Design review of the part shown in the three views and the two pictorial views. Dimensions are in mm from the part's minimum x, y and z. A direction names the side the tool comes from. Give positions to 0.01 mm unless a question says otherwise; leave off trailing zeros. Loops run counter-clockwise (first coordinate to the right, second up) from the corner with the lowest first, then second, coordinate; pieces in that order, holes last. Notation, with made-up numbers: (67, 24) - (79, 24) arc R26 ccw to (79, 40) - close; hole circle Ø1 at (43, 42.25). An arc over 180 degrees is marked (long way). Answer as a JSON object with one key per item and string values.
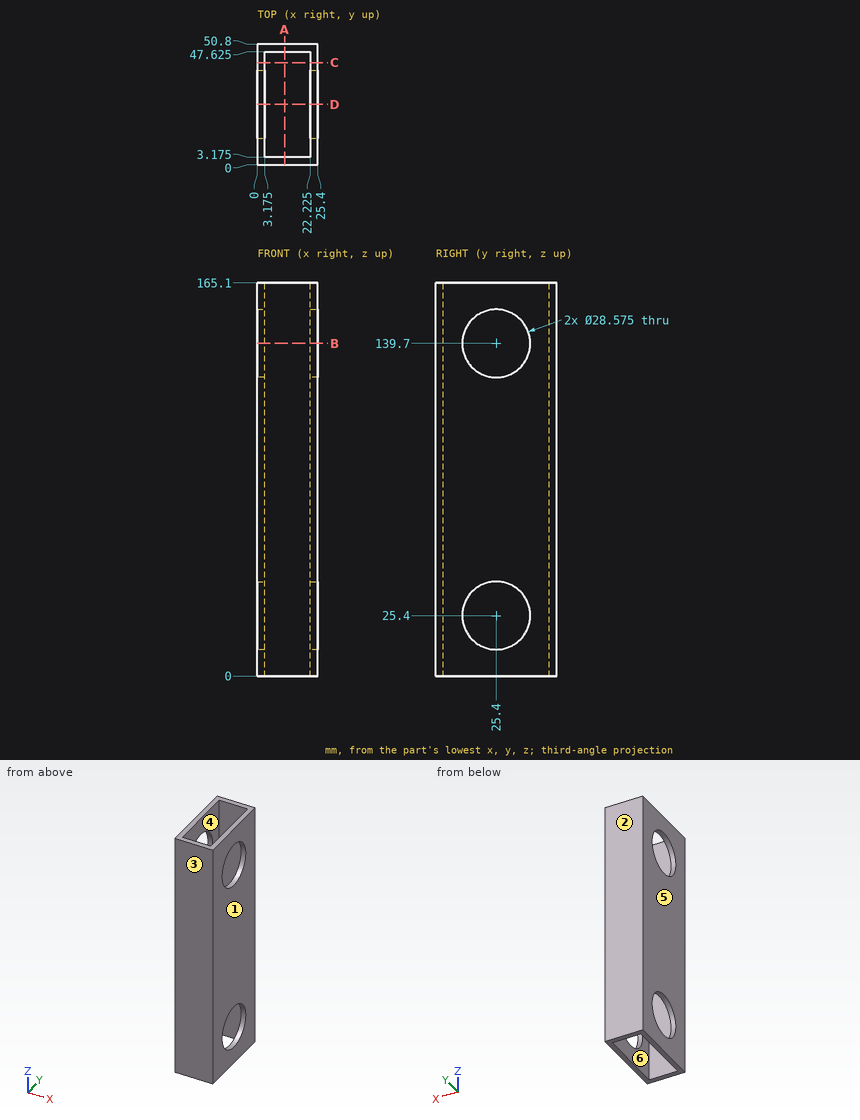
Q1. For the marked faces 5 and 6, list the 3-axis set-ups (+Z, -Z, +X, -X, +Y, -Y) from which the entire face can be reached by the end or side of a thin tool; tool diameter is ignored.
Results:
{"face 5": "+Z, -Z, -X, +Y, -Y", "face 6": "+Z, -Z"}
Q2. Consider section D-D, the plane y = 25.4. State the section outline as (x, z) points (1 decimal).
Results:
{"outline": "(0, 0) - (3.2, 0) - (3.2, 11.1) - (0, 11.1) - close; (0, 39.7) - (3.2, 39.7) - (3.2, 125.4) - (0, 125.4) - close; (0, 154) - (3.2, 154) - (3.2, 165.1) - (0, 165.1) - close; (22.2, 0) - (25.4, 0) - (25.4, 11.1) - (22.2, 11.1) - close; (22.2, 39.7) - (25.4, 39.7) - (25.4, 125.4) - (22.2, 125.4) - close; (22.2, 154) - (25.4, 154) - (25.4, 165.1) - (22.2, 165.1) - close"}
Q3. Consider section A-A, the plane x = 11.5. State the section outline as (y, z) points (3 decimals), plus the area to 3 significant figures.
Results:
{"outline": "(0, 0) - (3.175, 0) - (3.175, 165.1) - (0, 165.1) - close; (47.625, 0) - (50.8, 0) - (50.8, 165.1) - (47.625, 165.1) - close", "area": "1,050 mm^2"}
Q4. Consider section B-B, the plane z = 139.7. State the section outline as (x, y) points (1 decimal).
Results:
{"outline": "(0, 0) - (25.4, 0) - (25.4, 11.1) - (22.2, 11.1) - (22.2, 3.2) - (3.2, 3.2) - (3.2, 11.1) - (0, 11.1) - close; (0, 39.7) - (3.2, 39.7) - (3.2, 47.6) - (22.2, 47.6) - (22.2, 39.7) - (25.4, 39.7) - (25.4, 50.8) - (0, 50.8) - close"}
Q5. Consider section C-C, the plane y = 43. State the section outline as (x, z) points (3 decimals).
Results:
{"outline": "(0, 0) - (3.175, 0) - (3.175, 165.1) - (0, 165.1) - close; (22.225, 0) - (25.4, 0) - (25.4, 165.1) - (22.225, 165.1) - close"}
Q6. The part is to be moulded in two halves that separate along Y. For the marked faces 1, 2, 3 and 4, say which applies: +Y half, -Y half, draft (parallel to the pull), parting line (faces both ways), or undercut.
Results:
{"face 1": "draft", "face 2": "+Y half", "face 3": "-Y half", "face 4": "undercut"}
Q7. To check wall thickness, follow probe 1 along Y at (x, z) = (4.5, 59) (3 decimals); probe 2 along X at (y, z) = (28.5, 119.5) (3 decimals); probe 3 along Y at (x, z) = (1.8, 139.7). State the ranges of each line that lie inside material, in increasing order. Write a range as [from, to].
Results:
{"probe 1": "y = [0, 3.175], [47.625, 50.8]", "probe 2": "x = [0, 3.175], [22.225, 25.4]", "probe 3": "y = [0, 11.11], [39.69, 50.8]"}
